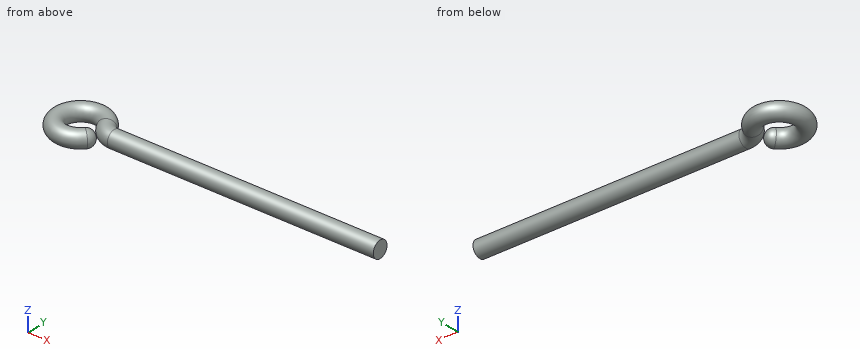
from build123d import *

# Parameters (mm, degrees)
SKETCH2_R           = 1
SKETCH3_R           = 1
BOSS_EXTRUDE1_DEPTH = 30
DOME1_FACE_RADIUS   = 1
DOME1_HEIGHT        = 1


with BuildPart() as part:
    # Sweep1: sweep along a path in Sketch1
    with BuildLine(Plane.XY) as sweep1_path:
        Line((0, 0), (-1.968871126, 0))
        ThreePointArc((-1.968871126, 0), (-3.022963679, 0.300326829), (-3.760483959, 1.111111111))
        ThreePointArc((-3.760483959, 1.111111111), (-8.482382241, 0.29627421), (-4.084888892, -1.606969024))
    # Sketch2 → Sweep1 (sweep)
    with BuildSketch(Plane(origin=(0, 0, 0), x_dir=(0, 0, -1), z_dir=(1, 0, 0))):
        Circle(SKETCH2_R)
    sweep(path=sweep1_path.line)

    # Sketch3 → Boss-Extrude1 (add)
    with BuildSketch(Plane(origin=(0, 0, 0), x_dir=(0, 0, -1), z_dir=(1, 0, 0))):
        with Locations(Location((0, 0, 0), (0, 0, 270))):
            Circle(SKETCH3_R)
    extrude(amount=BOSS_EXTRUDE1_DEPTH)

    # Dome1: a dome of height H over a round flat face of radius A is a cap of a sphere of radius (A * A + H * H) / (2 * H)
    dome1_r = (DOME1_FACE_RADIUS * DOME1_FACE_RADIUS + DOME1_HEIGHT * DOME1_HEIGHT) / (2 * DOME1_HEIGHT)
    dome1_base = Plane((-4.084888892, -1.606969024, 0), z_dir=(0.642787609687, 0.766044443119, 0))
    with Locations(dome1_base.offset(DOME1_HEIGHT - dome1_r)):
        dome1_ball = Sphere(dome1_r, mode=Mode.PRIVATE)
    add(split(dome1_ball, bisect_by=dome1_base, keep=Keep.TOP, mode=Mode.PRIVATE))


solid = part.part
Read the model definition and answer for the solid it produces. Units are mm, in the model's axes. Coordinates: 2 decimals unless noted, no trailing zeros. Order: outer loops, then holes, each group sorted by start corner. A loop starts at its lowest first (then second) coordinate and runs counter-clockwise, first axis right, second up. Notation, with made-up numbers: (81, -14.75) -> (106, -14.75) arc R6 cw to (106, -8.75) -> close; hole circle Ø7 at (0.25, -10). An arc over 180 degrees is marked (long way). Answer as a JSON object with one key per item and string values.
1) A cutting plane is placed at A-A, the plane x = 6. Determine the outline of the cut face in (y, z), plus the area to 3 significant figures.
Model answer:
{"outline": "circle Ø2 at (0, 0)", "area": "3.14 mm²"}
2) Consider line 1 along X through (y, z) = (-1, 0.55); line 2 along Z through (x, y) = (-6.5, -2.5); line 3 along Y through (x, z) = (-3.5, 0). Determine where each line is inside the solid, lowest interval first. Write a range as from..to.
Model answer:
{"line 1": "x = -9.18..-7.33, -4.66..-3.51", "line 2": "z = -1..1", "line 3": "y = -2.45..-0.8, -0.58..2.45"}
3) A cutting plane is placed at B-B, the plane z = -0.55. Determine the outline of the cut face in (x, y).
Model answer:
{"outline": "(-4.72, -1.07) arc R1.66 cw (long way) to (-4.51, 0.74) arc R2.84 ccw to (-1.97, -0.84) -> (30, -0.84) -> (30, 0.84) -> (-1.97, 0.84) arc R1.16 cw to (-3.01, 1.48) arc R3.34 ccw (long way) to (-3.45, -2.14) arc R0.84 ccw to start"}
